Geometry check sheet. Reference: the model listing, model coordinates, mm. Face numbers are marked on the shaded views. A direction names the side the tool comes from. Round coordinates to 2 decimals unless told otherwise and drop trailing zeros. Order: outer loops, then holes, each group sorted by start corner. A loop starts at its lowest first (then second) coordinate and runs counter-clockwise, first axis right, second up.
(1) Draft check along Y on the marked faces 4, 5 and 6. Enter one of: pulls with the +Y half, pulls with the -Y half, needs draft (parallel to the pull), parting line crosses it, or undercut.
(2) Cross-section at A-A on z = 14.1. Enter the section's corners in (x, y), and give its area (3 significant figures).
(3) Cross-section at B-B on y = 24. Enter the section's corners in (x, z).
(4) Gauge pin test, flat ends, axial feed: P1, Ø15, axis at x = -5.5, z = 9, coming from the +Y side; P2, Ø10, axis at x = 28, y = 21, coming from the +Z side; P3, Ø8, axis at x = -20, z = 9, coming from the +Y side; P4, Ø0.9, axis at y = 1.5, z = 7, coming from the +X side. Record the tip position at first contact, or that the pin passes through.
(5) Set-up check for the marked faces 1, 2 and 3: record each of +Z, -Z, +X, -X, +Y, -Y from which the full face is reachable in a straight line by a thin tool's end or side.
(6) Cross-section at C-C on x = 31.5. Enter the section's corners in (y, z), and give its area (3 significant figures).
(7) Thickness scan on L1, parallel to X at y = 28, z = 3.5; L2, parallel to X at y = 1.9, z = 6.1; L3, parallel to Z at x = 32, y = 9. Record the ranges inside material, lowest first.
(8) Cross-section at D-D on z = 6.1. Count the separate pieces of the cut face and the enclosed holes in it, and give its area (3 significant figures).
from build123d import *

# Parameters (mm, degrees)
SKETCH1_W           = 28.2
SKETCH1_H           = 19
BOSS_EXTRUDE1_DEPTH = 3
SKETCH2_R           = 2.1
BOSS_EXTRUDE2_DEPTH = 6
BOSS_EXTRUDE3_DEPTH = 3
FILLET1_R           = 2
SKETCH4_R           = 2.1
BOSS_EXTRUDE4_DEPTH = 2
BOSS_EXTRUDE5_DEPTH = 16
FILLET2_R           = 2
SHELL1_START        = -4
SHELL1_DEPTH        = 12
SKETCH6_W           = 38.395963329
SKETCH6_H           = 16
SKETCH6_W_2         = 34.354282979
SKETCH6_H_2         = 12
SKETCH6_W_3         = 24.354282979
BOSS_EXTRUDE6_DEPTH = 1
CHAMFER1_SIZE       = 2.887134603
CHAMFER1_SIZE_2     = 3


with BuildPart() as part:
    # Sketch1 → Boss-Extrude1 (new body)
    with BuildSketch(Plane(origin=(0, 0, 0), x_dir=(1, 0, 0), z_dir=(0, 1, 0))):
        with Locations((0, -9.5)):
            Rectangle(SKETCH1_W, SKETCH1_H)
        with BuildLine():
            Line((-9.34985398, -7.708693331), (-8, -8.841355308))
            Line((-8, -8.841355308), (-6.65014602, -7.708693331))
            ThreePointArc((-6.65014602, -7.708693331), (-8, -4), (-9.34985398, -7.708693331))
        make_face(mode=Mode.SUBTRACT)
        with BuildLine():
            Line((-1.34985398, -15.708693331), (0, -16.841355308))
            Line((0, -16.841355308), (1.34985398, -15.708693331))
            ThreePointArc((1.34985398, -15.708693331), (0, -12), (-1.34985398, -15.708693331))
        make_face(mode=Mode.SUBTRACT)
        with BuildLine():
            Line((6.65014602, -7.708693331), (8, -8.841355308))
            Line((8, -8.841355308), (9.34985398, -7.708693331))
            ThreePointArc((9.34985398, -7.708693331), (8, -4), (6.65014602, -7.708693331))
        make_face(mode=Mode.SUBTRACT)
    extrude(amount=BOSS_EXTRUDE1_DEPTH)

    # Sketch2 → Boss-Extrude2 (add)
    with BuildSketch(Plane(origin=(0, 0, 0), x_dir=(-1, 0, 0), z_dir=(0, 0, -1))):
        Polygon((-14.1, 0), (14.1, 0), (12.1, 50.1), (-12.1, 50.1), align=None)
        with Locations((-8, 46)):
            Circle(SKETCH2_R, mode=Mode.SUBTRACT)
        with Locations((8, 46)):
            Circle(SKETCH2_R, mode=Mode.SUBTRACT)
    extrude(amount=BOSS_EXTRUDE2_DEPTH)

    # Sketch3 → Boss-Extrude3 (add, symmetric)
    with BuildSketch(Plane(origin=(0, 0, 0), x_dir=(0, 0, -1), z_dir=(1, 0, 0))):
        Polygon((0, 3), (-10, 3), (0, 38), align=None)
    extrude(amount=BOSS_EXTRUDE3_DEPTH, both=True)

    # Fillet1
    fillet1_edges = [part.edges().sort_by_distance(p)[0] for p in [
        (12.1, 50.1, -3),
        (-12.1, 50.1, -3),
        (14.1, 1.5, 19),
        (-14.1, 1.5, 19),
    ]]
    fillet(fillet1_edges, radius=FILLET1_R)

    # Sketch4 → Boss-Extrude4 (add)
    with BuildSketch(Plane.XY):
        with BuildLine():
            Line((-10.178247335, 50.1), (10.178247335, 50.1))
            ThreePointArc((10.178247335, 50.1), (11.563968527, 49.54214312), (12.176655618, 48.179776778))
            Line((12.176655618, 48.179776778), (12.459281437, 41.1))
            Line((12.459281437, 41.1), (-12.459281437, 41.1))
            Line((-12.459281437, 41.1), (-12.176655618, 48.179776778))
            ThreePointArc((-12.176655618, 48.179776778), (-11.563968527, 49.54214312), (-10.178247335, 50.1))
        make_face()
        with Locations(Location((-8, 46, 0), (0, 0, 180))):
            Circle(SKETCH4_R, mode=Mode.SUBTRACT)
        with Locations(Location((8, 46, 0), (0, 0, 180))):
            Circle(SKETCH4_R, mode=Mode.SUBTRACT)
    extrude(amount=BOSS_EXTRUDE4_DEPTH)


with BuildPart() as body_2:
    # Sketch5 → Boss-Extrude5 (new body)
    with BuildSketch(Plane(origin=(0, 0, -6), x_dir=(-1, 0, 0), z_dir=(0, 0, -1))):
        Polygon((12.513173653, 39.75), (50.513173653, 45.25), (50.513173653, 4.75), (12.513173653, 4.75), align=None)
    extrude(amount=-BOSS_EXTRUDE5_DEPTH)

    # Fillet2
    fillet2_edges = [body_2.edges().sort_by_distance(p)[0] for p in [
        (-50.513173653, 4.75, 2),
    ]]
    fillet(fillet2_edges, radius=FILLET2_R)

    # Shell1: read off the stored shape, not the designer's step
    # Shell1 outline → Shell1 (cut)
    with BuildSketch(Plane.XY.offset(SHELL1_START)):
        Polygon((-48.513173653, 44.960526316), (-48.513173653, 6.75), (-14.513173653, 6.75), (-14.513173653, 40.039473684), align=None)
    extrude(amount=SHELL1_DEPTH, mode=Mode.SUBTRACT)

    # Sketch6 → Boss-Extrude6 (add)
    # profile 1 of 2: a face of its own
    with BuildSketch(Plane(origin=(5.378481599, 37.160418319, 0), x_dir=(0.9896873708806833, -0.14324422473273113, 0), z_dir=(0.14324422473273113, 0.9896873708806833, 0))):
        with Locations((-37.276069531, -2)):
            Rectangle(SKETCH6_W, SKETCH6_H)
        with Locations((-37.276069531, -2)):
            Rectangle(SKETCH6_W_2, SKETCH6_H_2, mode=Mode.SUBTRACT)
    # profile 2 of 2: a face of its own
    with BuildSketch(Plane(origin=(5.378481599, 37.160418319, 0), x_dir=(0.9896873708806833, -0.14324422473273113, 0), z_dir=(0.14324422473273113, 0.9896873708806833, 0))):
        with Locations((-42.276069531, -2)):
            Rectangle(SKETCH6_W_3, SKETCH6_H_2)
    extrude(amount=BOSS_EXTRUDE6_DEPTH)


with BuildPart() as body_3:
    # Mirror2: mirrored copy
    add(body_2.part.mirror(Plane(origin=(0, 0, 0), x_dir=(0, 0, 1), z_dir=(1, 0, 0))))


with BuildPart() as part_1:
    add(part.part)

    # Combine1: read off the stored shape, not the designer's step
    # Combine1: union body 3, body 2
    add(body_3.part)
    add(body_2.part)

    # Chamfer1
    # the kernel refuses this chamfer: 3, 2.887134603 mm, written as the material it adds along each edge
    with BuildSketch(Plane(origin=(-13.910379242, 4.75, -6), x_dir=(-0.039888388883066415, -0.9992041415207972, 0), z_dir=(0, 0, 1))) as chamfer1_piece_1:
        Polygon((CHAMFER1_SIZE, 0), (CHAMFER1_SIZE_2 * 0.0398883888831, -CHAMFER1_SIZE_2 * 0.999204141521), (0, 0), align=None)
    extrude(amount=6)
    with BuildSketch(Plane(origin=(13.910379242, 4.75, -6), x_dir=(0.039888388883066304, -0.9992041415207972, 0), z_dir=(0, 0, 1))) as chamfer1_piece_2:
        Polygon((CHAMFER1_SIZE, 0), (CHAMFER1_SIZE_2 * 0.0398883888831, CHAMFER1_SIZE_2 * 0.999204141521), (0, 0), align=None)
    extrude(amount=6)


solid = part_1.part
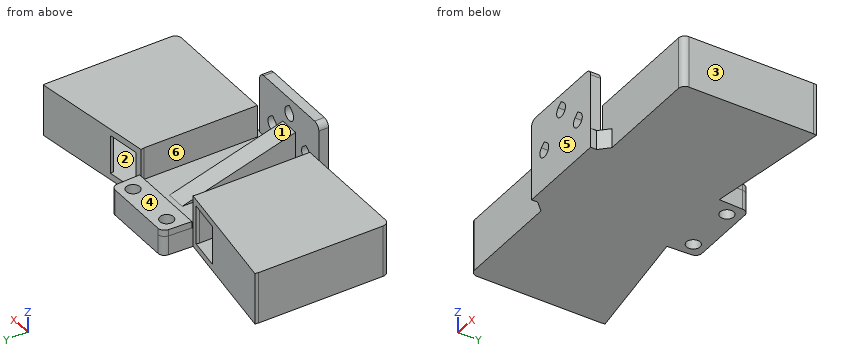
Found:
1. face 4: needs draft
1. face 5: pulls with the -Y half
1. face 6: undercut
2. outline: (-14.1, 0) - (-2.1, 0) - (-2.1, 3) - (-14.1, 3) - close; (2.1, 0) - (14.1, 0) - (14.1, 3) - (2.1, 3) - close
2. area: 72.0 mm2
3. outline: (-50.51, -6) - (50.51, -6) - (50.51, 10) - (12.51, 10) - (12.51, 0) - (3, 0) - (3, 4) - (-3, 4) - (-3, 0) - (-12.51, 0) - (-12.51, 10) - (-50.51, 10) - close; hole (-48.51, -4) - (-14.51, -4) - (-14.51, 8) - (-48.51, 8) - close; hole (14.51, -4) - (48.51, -4) - (48.51, 8) - (14.51, 8) - close
4. P1: stops at y = 50.1
4. P2: stops at z = 10
4. P3: stops at y = 42.42
4. P4: stops at x = 14.1
5. face 1: +Z
5. face 2: none
5. face 3: +Z, -Z, +X, +Y, -Y
6. outline: (4.75, -6) - (43.51, -6) - (43.51, 10) - (4.75, 10) - close; hole (6.75, -4) - (42.5, -4) - (42.5, 8) - (6.75, 8) - close
6. area: 191 mm2
7. L1: x = -50.51 to -48.51, -14.51 to -12.51, 12.51 to 14.51, 48.51 to 50.51
7. L2: x = -14.1 to -10.1, -5.9 to 5.9, 10.1 to 14.1
7. L3: z = -6 to -4, 8 to 10
8. separate pieces: 5
8. enclosed holes: 0
8. area: 634 mm2
